```python
from build123d import *

# Parameters (mm, degrees)
F0_R     = 3
F1_DEPTH = 3
F2_SIZE  = 2
F3_SIZE  = 0.5
F4_SIZE  = 0.5


with BuildPart() as f1:
    # F0 (on Front) → F1 (new body)
    with BuildSketch(Plane.XZ):
        with BuildLine():
            ThreePointArc((5, 0), (15, -10), (25, 0))
            ThreePointArc((25, 0), (0, 25), (-25, 0))
            ThreePointArc((-25, 0), (-23.515691, -5.242423), (-19.5034, -8.928571))
            ThreePointArc((-19.5034, -8.928571), (-12.938924, -14.570541), (-9.766986, -22.624297))
            Line((-9.766986, -22.624297), (-5.491523, -54.734824))
            ThreePointArc((-5.491523, -54.734824), (-3.665561, -58.303294), (0, -59.925571))
            Line((0, -59.925571), (0, -5))
            ThreePointArc((0, -5), (-3.535534, 3.535534), (5, 0))
        make_face()
        with Locations((-15, 0)):
            Circle(F0_R, mode=Mode.SUBTRACT)
        with Locations((15, 0)):
            Circle(F0_R, mode=Mode.SUBTRACT)
    extrude(amount=F1_DEPTH)

    # F2
    f2_edges = [f1.edges().sort_by_distance(p)[0] for p in [
        (0, -3, -32.462785),
    ]]
    chamfer(f2_edges, length=F2_SIZE)

    # F3
    f3_edges = [f1.edges().sort_by_distance(p)[0] for p in [
        (-18, -3, 0),
    ]]
    chamfer(f3_edges, length=F3_SIZE)

    # F4
    f4_edges = [f1.edges().sort_by_distance(p)[0] for p in [
        (12, -3, 0),
    ]]
    chamfer(f4_edges, length=F4_SIZE)


solid = f1.part
```
Geometry check sheet. Reference: the model listing, model coordinates, mm. Coordinates: 2 decimals unless noted, no trailing zeros. Loops run counter-clockwise (first coordinate to the right, second up) from the corner with the lowest first, then second, coordinate; pieces in that order, holes last. Notation, with made-up numbers: (39, 30.25) -> (51, 30.25) arc R20 cw to (51, 38.25) -> close; hole circle Ø2 at (15.25, 54). An arc over 180 degrees is marked (long way). Put each result on its own line as item: value.
1) Release check for a two-part mould opening along Z. For faces 1 (the cylindrical face through (-4, -1, 3)), 2 (the cylindrical face through (-3.71, -1.48, -58.26)), 3 (the flat face through (5, -3, 2)), 4 (the cylindrical face through (12, -1, 0)) record: released by +Z, released by -Z, zero draft, split by the parting line, or undercut.
Result set:
face 1: undercut
face 2: released by -Z
face 3: zero draft
face 4: undercut
2) Cross-section at B-B on x = 15. Record the boundary of the cut face in (y, z), plus the area to 4 significant figures.
Result set:
outline: (-3, -10) -> (0, -10) -> (0, -3) -> (-2.5, -3) -> (-3, -3.5) -> close; (-3, 3.5) -> (-2.5, 3) -> (0, 3) -> (0, 20) -> (-3, 20) -> close
area: 71.75 mm^2
3) Gauge pin test, flat ends, axial feed: pin 1 Ø1.5 at (y, z) = (-2.5, -7.5) entering from -X; pin 2 Ø1 at (y, z) = (-0.5, 1) entering from +X (3 decimals). Record the tip position at first contact, or that the pin passes through.
Result set:
pin 1: stops at x = -22.38
pin 2: stops at x = 24.995
4) Cross-section at C-C on y = -1.75. Record the boundary of the cut face in (x, z).
Result set:
outline: (-25, 0) arc R10 ccw to (-19.5, -8.93) arc R18 cw to (-9.77, -22.62) -> (-5.49, -54.73) arc R6 ccw to (-0.75, -59.82) -> (-0.75, -4.94) arc R5 cw (long way) to (5, 0) arc R10 ccw to (25, 0) arc R25 ccw to start; hole circle Ø6 at (-15, 0); hole circle Ø6 at (15, 0)
5) Thickness scan on line 1 (Z direction, x = 0, y = -2.2); line 2 (Z direction, x = -17, y = -1.45); line 3 (Z direction, x = -3, y = -2). Record the ranges inside material, lowest first.
Result set:
line 1: z = 5 to 25
line 2: z = -10.46 to -2.24, 2.24 to 18.33
line 3: z = -58.85 to -4, 4 to 24.82
6) Cross-section at A-A on z = -6. Record the boundary of the cut face in (x, y), plus the area to 3 significant figures.
Result set:
outline: (-23, -3) -> (-2, -3) -> (0, -1) -> (0, 0) -> (-23, 0) -> close; (7, -3) -> (23, -3) -> (23, 0) -> (7, 0) -> close
area: 115 mm^2
7) Cross-section at D-D on z = -23.5. Record the boundary of the cut face in (x, y).
Result set:
outline: (-9.65, -3) -> (-2, -3) -> (0, -1) -> (0, 0) -> (-9.65, 0) -> close
